```python
from build123d import *

# Parameters (mm, degrees)
BOSS_EXTRUDE1_DEPTH = 6.35
SKETCH2_R           = 104.764774547
CUT_EXTRUDE1_DEPTH  = 243.550051536


with BuildPart() as part:
    # Sketch1 → Boss-Extrude1 (new body)
    with BuildSketch(Plane.XY):
        with BuildLine():
            Line((-158.75, 171.45), (158.75, 171.45))
            ThreePointArc((158.75, 171.45), (167.730256121, 167.730256121), (171.45, 158.75))
            Line((171.45, 158.75), (171.45, -158.75))
            ThreePointArc((171.45, -158.75), (167.730256121, -167.730256121), (158.75, -171.45))
            Line((158.75, -171.45), (-158.75, -171.45))
            ThreePointArc((-158.75, -171.45), (-167.730256121, -167.730256121), (-171.45, -158.75))
            Line((-171.45, -158.75), (-171.45, 158.75))
            ThreePointArc((-171.45, 158.75), (-167.730256121, 167.730256121), (-158.75, 171.45))
        make_face()
    extrude(amount=BOSS_EXTRUDE1_DEPTH)

    # Sketch2 → Cut-Extrude1 (cut, through all)
    with BuildSketch(Plane.XY.offset(6.35)):
        Circle(SKETCH2_R)
    extrude(amount=-CUT_EXTRUDE1_DEPTH, mode=Mode.SUBTRACT)


solid = part.part
```
For this review, take the finished solid that the model builds, in its own axes (mm). Coordinates: 2 decimals unless noted, no trailing zeros. Loops run counter-clockwise (first coordinate to the right, second up) from the corner with the lowest first, then second, coordinate; pieces in that order, holes last.
1. Add section A-A, the plane x = 0. Give the boundary of the cut face in (y, z), then the cut area to 3 significant figures.
2. For line 1 (Y direction, x = 0, z = 4.25); line 2 (Y direction, x = -13, z = 2); line 3 (X direction, y = -87, z = 4.5), list the stretches that pass through material, from the lowest coordinate up.
3. Add section C-C, the plane z = 5. Give the boundary of the cut face in (x, y).
4. Mouldability with a two-part tool opening along Y and no side actions: class faces 1 (the cylindrical face through (-167.63, -167.83, 3.13)), 2 (the flat face through (79, 79, 0)), 3 (the cylindrical face through (167.63, 167.83, 3.13)), 4 (the cylindrical face through (-22.711, -102.274, 3.219)) as +Y half, -Y half, draft (parallel to the pull), parting line (faces both ways), or undercut.
Result:
1. outline: (-171.45, 0) - (-104.76, 0) - (-104.76, 6.35) - (-171.45, 6.35) - close; (104.76, 0) - (171.45, 0) - (171.45, 6.35) - (104.76, 6.35) - close
1. area: 847 mm2
2. line 1: y = -171.45 to -104.76, 104.76 to 171.45
2. line 2: y = -171.45 to -103.96, 103.96 to 171.45
2. line 3: x = -171.45 to -58.37, 58.37 to 171.45
3. outline: (-171.45, -158.75) arc R12.7 ccw to (-158.75, -171.45) - (158.75, -171.45) arc R12.7 ccw to (171.45, -158.75) - (171.45, 158.75) arc R12.7 ccw to (158.75, 171.45) - (-158.75, 171.45) arc R12.7 ccw to (-171.45, 158.75) - close; hole circle Ø209.53 at (0, 0)
4. face 1: -Y half
4. face 2: draft
4. face 3: +Y half
4. face 4: undercut
